CAD build for the part. Positions are in the model's coordinates, mm. Round coordinates to 2 decimals unless told otherwise and drop trailing zeros. Write each loop counter-clockwise with the first axis right and the second up, starting at its lowest first coordinate (ties: lowest second). Pieces come first, ordered by that corner, then holes. Notation, with made-up numbers: (20.5, 27.25) - (53.5, 27.25) arc R29 ccw to (53.5, 53.25) - close; hole circle Ø3 at (2.5, 69.5). An arc over 180 degrees is marked (long way). Answer in a Markdown table with one row per item.
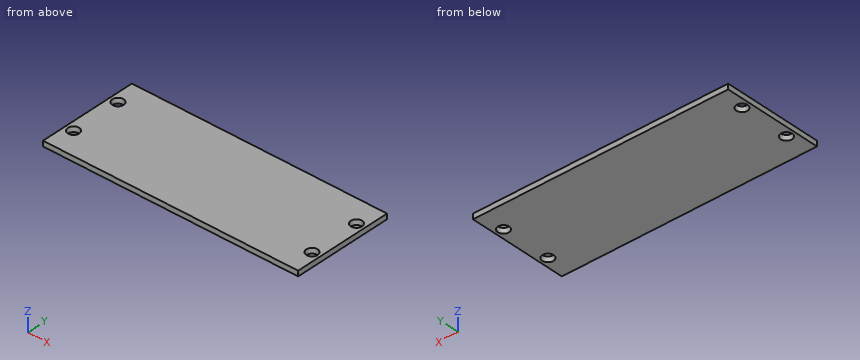
```python
from build123d import *

# Parameters (mm, degrees)
F0_W     = 146.05
F0_H     = 57.15
F0_R     = 3.24
F1_DEPTH = 3


# Not quite as in the source:
# - ends of sketch curves that miss each other by under 0.0002 mm in the source are joined


with BuildPart() as f1:
    # F0 (on Top) → F1 (new body)
    with BuildSketch(Plane.XY):
        Rectangle(F0_W, F0_H)
        with Locations((-68.262, -14.287)):
            Circle(F0_R, mode=Mode.SUBTRACT)
        with Locations((68.262, -14.287)):
            Circle(F0_R, mode=Mode.SUBTRACT)
        with Locations((-68.262, 14.287)):
            Circle(F0_R, mode=Mode.SUBTRACT)
        with BuildLine():
            ThreePointArc((-68.262, 7.937), (-61.912, 14.287), (-68.262, 20.637))
            Line((-68.262, 20.637), (-72.225, 20.637))
            Line((-72.225, 20.637), (-72.225, 27.775))
            Line((-72.225, 27.775), (72.225, 27.775))
            Line((72.225, 27.775), (72.225, 20.636958))
            Line((72.225, 20.636958), (69.238962, 20.636958))
            ThreePointArc((69.238962, 20.636958), (62.9120417914, 14.2639619992), (69.2850380008, 7.9370417914))
            Line((69.2850380008, 7.9370417914), (72.225, 7.937042))
            Line((72.225, 7.937042), (72.225, -7.937576))
            Line((72.225, -7.937576), (68.176478, -7.937576))
            ThreePointArc((68.176478, -7.937576), (61.9125759326, -14.3725220009), (68.3475220009, -20.6364240674))
            Line((68.3475220009, -20.6364240674), (72.225, -20.636424))
            Line((72.225, -20.636424), (72.225, -27.775))
            Line((72.225, -27.775), (-72.225, -27.775))
            Line((-72.225, -27.775), (-72.225, -20.636871))
            Line((-72.225, -20.636871), (-69.221508, -20.636871))
            ThreePointArc((-69.221508, -20.636871), (-62.9121291038, -14.2465080007), (-69.3024919993, -7.9371291038))
            Line((-69.3024919993, -7.9371291038), (-72.225, -7.937129))
            Line((-72.225, -7.937129), (-72.225, 7.937))
            Line((-72.225, 7.937), (-68.262, 7.937))
        make_face(mode=Mode.SUBTRACT)
        with Locations((68.262, 14.287)):
            Circle(F0_R, mode=Mode.SUBTRACT)
        with BuildLine():
            Line((-72.225, 20.637), (-68.262, 20.637))
            ThreePointArc((-68.262, 20.637), (-61.912, 14.287), (-68.262, 7.937))
            Line((-68.262, 7.937), (-72.225, 7.937))
            Line((-72.225, 7.937), (-72.225, -7.937129))
            Line((-72.225, -7.937129), (-69.302492, -7.937129))
            ThreePointArc((-69.302492, -7.937129), (-62.9121291038, -14.2465080007), (-69.2215080007, -20.6368708962))
            Line((-69.2215080007, -20.6368708962), (-72.225, -20.636871))
            Line((-72.225, -20.636871), (-72.225, -27.775))
            Line((-72.225, -27.775), (72.225, -27.775))
            Line((72.225, -27.775), (72.225, -20.636424))
            Line((72.225, -20.636424), (68.347522, -20.636424))
            ThreePointArc((68.347522, -20.636424), (61.9125759326, -14.3725220009), (68.1764779991, -7.9375759326))
            Line((68.1764779991, -7.9375759326), (72.225, -7.937576))
            Line((72.225, -7.937576), (72.225, 7.937042))
            Line((72.225, 7.937042), (69.285038, 7.937042))
            ThreePointArc((69.285038, 7.937042), (62.9120417914, 14.2639619992), (69.2389619992, 20.6369582086))
            Line((69.2389619992, 20.6369582086), (72.225, 20.636958))
            Line((72.225, 20.636958), (72.225, 27.775))
            Line((72.225, 27.775), (-72.225, 27.775))
            Line((-72.225, 27.775), (-72.225, 20.637))
        make_face()
    extrude(amount=F1_DEPTH)


solid = f1.part
```
Q1. Drill centre lines: line 1 (X direction, y = -14, z = 1.45) (3 decimals); line 2 (X direction, y = -15.5, z = 0.55) (3 decimals); line 3 (Y direction, x = 67.5, z = 1.05) (3 decimals). Where is each one in solid material? Low to high.
Computed:
| item | result |
|---|---|
| line 1 | x = -73.025 to -71.489, -65.035 to 65.035, 71.489 to 73.025 |
| line 2 | x = -73.025 to -71.266, -65.258 to 65.258, 71.266 to 73.025 |
| line 3 | y = -28.575 to -17.436, -11.138 to 11.138, 17.436 to 28.575 |
Q2. Saw through at A-A on z = 0.7. List the corners of the cut face in (x, y) (3 decimals), then the cut area to 3 significant figures.
Computed:
| item | result |
|---|---|
| outline | (-73.025, -28.575) - (73.025, -28.575) - (73.025, 28.575) - (-73.025, 28.575) - close; hole circle Ø6.48 at (-68.262, -14.287); hole circle Ø6.48 at (-68.262, 14.287); hole circle Ø6.48 at (68.262, -14.287); hole circle Ø6.48 at (68.262, 14.287) |
| area | 8,210 mm2 |
Q3. Flat gauge pin, fed straight in: pin 1 (4 mm diameter, centred on x = -68.262, y = -14.287, fed in from -Z). Where does the tip first touch, or does it go through?
Computed:
| item | result |
|---|---|
| pin 1 | passes through |
